For this review, use the dimensioned drawing (mm, ordinates from the lowest corner) and the shaded views. A direction names the side the tool comes from. Coordinates: 2 decimals unless noted, no trailing zeros. Write each loop counter-clockwise with the first axis right and the second up, starting at its lowest first coordinate (ties: lowest second). Pieces come first, ordered by that corner, then holes. Notation, with made-up numbers: (65, 88.5) - (120, 88.5) arc R18 ccw to (120, 101.5) - close; hole circle Ø7 at (-15.5, 10.5). An arc over 180 degrees is marked (long way). Use one line per item in the form item = value. Start each with the question number.
1) We need section C-C (y = 28). Give the boundary of the cut face in (x, z), plus the area to 3 significant figures.
2) We need section A-A (x = 28). Give the boundary of the cut face in (y, z), plus the area to 3 significant figures.
3) Insertion check: P1, Ø4.5, axis at x = 3.5, z = 32.5, coming from the +Y side; P2, Ø2.5, axis at x = 6.5, z = 12.5, coming from the -Y side; P3, Ø4.5, axis at y = 49.5, z = 17.5, coming from the -X side. Each pin has a flat end and moves straight along its axis. Give the tip position at first contact, or say it passes through.
4) We need section B-B (z = 37.5). Give the boundary of the cut face in (x, y).
5) We need section D-D (y = 37). Give the boundary of the cut face in (x, z), plus the area to 3 significant figures.
6) Tool access review of the marked faces 1, 2 and 3: name each direction out of +Z, -Z, +X, -X, +Y, -Y from which nothing blocks a thin tool from reaching the whole face with its end or side.
7) For L1, parallel to Y at x = 4.5, z = 51.55; L2, parallel to Y at x = 4, z = 50; L3, parallel to X at y = 51, z = 49, list the stretches that pass through material, from the lowest coordinate up. Write a range as from..to.
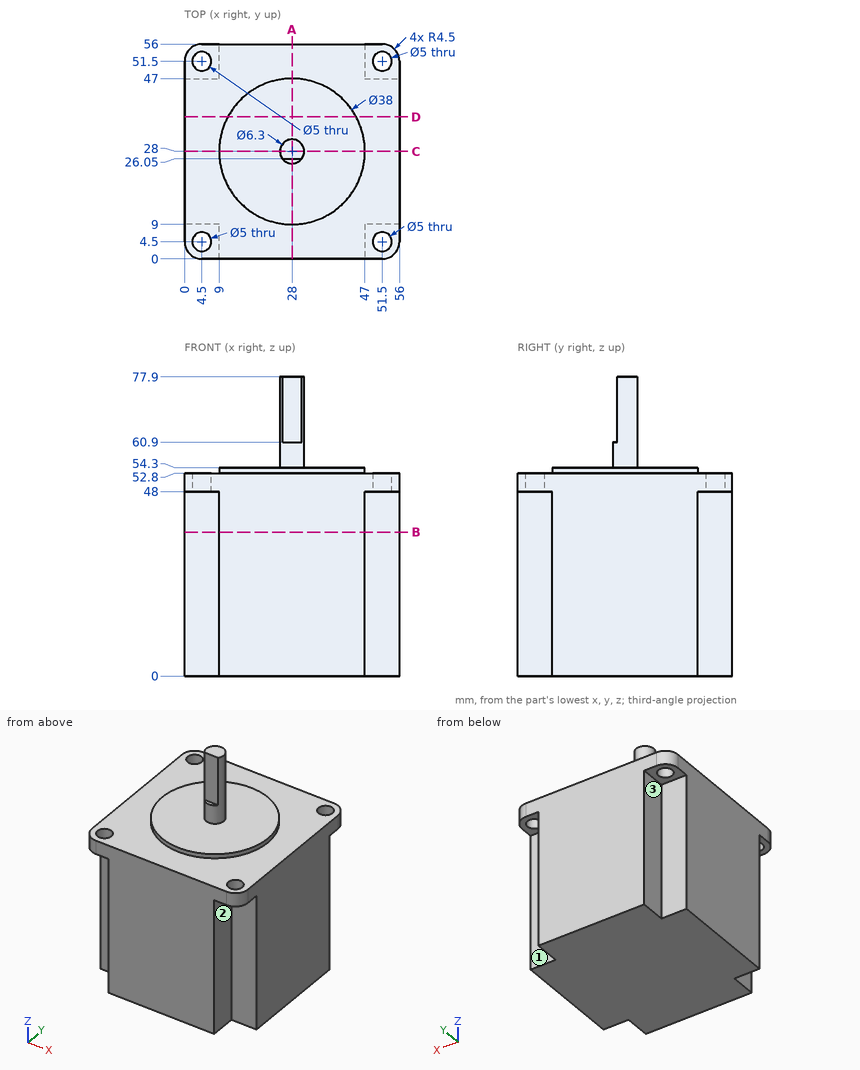
Determined:
q1.outline = (0, 0) - (56, 0) - (56, 52.8) - (47, 52.8) - (47, 54.3) - (31.15, 54.3) - (31.15, 77.9) - (24.85, 77.9) - (24.85, 54.3) - (9, 54.3) - (9, 52.8) - (0, 52.8) - close
q1.area = 3,160 mm²
q2.outline = (0, 0) - (56, 0) - (56, 52.8) - (47, 52.8) - (47, 54.3) - (31.15, 54.3) - (31.15, 77.9) - (26.05, 77.9) - (26.05, 60.9) - (24.85, 60.9) - (24.85, 54.3) - (9, 54.3) - (9, 52.8) - (0, 52.8) - close
q2.area = 3,140 mm²
q3.P1 = 47
q3.P2 = 9
q3.P3 = 9
q4.outline = (0, 9) - (9, 9) - (9, 0) - (47, 0) - (47, 9) - (56, 9) - (56, 47) - (47, 47) - (47, 56) - (9, 56) - (9, 47) - (0, 47) - close
q5.outline = (0, 0) - (56, 0) - (56, 52.8) - (44.73, 52.8) - (44.73, 54.3) - (11.27, 54.3) - (11.27, 52.8) - (0, 52.8) - close
q5.area = 3,010 mm²
q6.face_1 = -Z, +X, +Y
q6.face_2 = -Z, +X, -Y
q6.face_3 = -Z, -X, +Y
q7.L1 = 0..2, 7..49, 54..56
q7.L2 = 0.03..2.05, 6.95..49.05, 53.95..55.97
q7.L3 = 0..2.05, 6.95..49.05, 53.95..56
